Geometry: final body of the model. Coordinates: model frame, mm. Face numbers are marked on the shaded views. A direction names the side the tool comes from. Give positions to 0.01 mm unless a question says otherwise; leave off trailing zeros. Write each loop counter-clockwise with the first axis right and the second up, starting at its lowest first coordinate (ties: lowest second). Pieces come first, ordered by that corner, then holes.
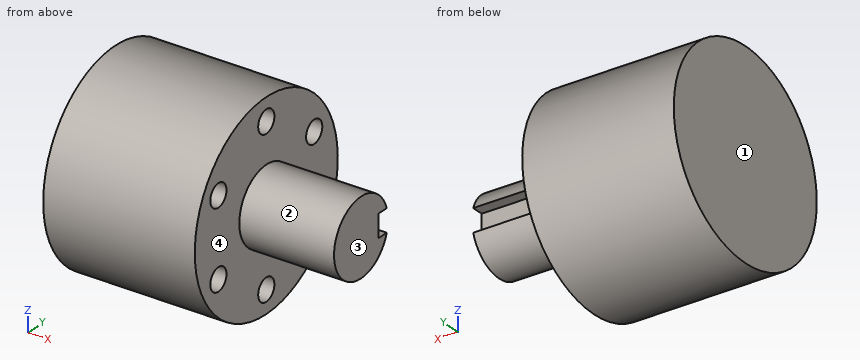
from build123d import *

# Parameters (mm, degrees)
SKETCH_1_R          = 13.25
EXTRUDE_1_DEPTH     = 20
SKETCH_2_R          = 1.5
CUT_EXTRUDE_1_DEPTH = 5
SKETCH_3_R          = 5
EXTRUDE_2_DEPTH     = 12.5
CUT_EXTRUDE_START   = -10
CUT_EXTRUDE_2_DEPTH = 10


with BuildPart() as part:
    # 草图1 → 凸台-拉伸1 (new body)
    with BuildSketch(Plane(origin=(0, 0, 0), x_dir=(0, 0, -1), z_dir=(1, 0, 0))):
        Circle(SKETCH_1_R)
    extrude(amount=EXTRUDE_1_DEPTH)

    # 草图2 → 切除-拉伸1 (cut)
    with BuildSketch(Plane(origin=(20, 0, 0), x_dir=(0, 0, -1), z_dir=(1, 0, 0))):
        with Locations((10.25, 0)):
            Circle(SKETCH_2_R)
        with Locations((5.125, -8.876760389)):
            Circle(SKETCH_2_R)
        with Locations((-5.125, -8.876760389)):
            Circle(SKETCH_2_R)
        with Locations((-10.25, 0)):
            Circle(SKETCH_2_R)
        with Locations((-5.125, 8.876760389)):
            Circle(SKETCH_2_R)
        with Locations((5.125, 8.876760389)):
            Circle(SKETCH_2_R)
    extrude(amount=-CUT_EXTRUDE_1_DEPTH, mode=Mode.SUBTRACT)

    # 草图3 → 凸台-拉伸2 (add)
    with BuildSketch(Plane(origin=(20, 0, 0), x_dir=(0, 0, -1), z_dir=(1, 0, 0))):
        Circle(SKETCH_3_R)
    extrude(amount=EXTRUDE_2_DEPTH)

    # 草图4 → 切除-拉伸2 (cut)
    with BuildSketch(Plane(origin=(32.5, 0, 0), x_dir=(0, 0, -1), z_dir=(1, 0, 0)).offset(CUT_EXTRUDE_START)):
        with BuildLine():
            Line((-1.5, 3.2), (1.5, 3.2))
            Line((1.5, 3.2), (1.5, 4.769696007))
            ThreePointArc((1.5, 4.769696007), (0, 5), (-1.5, 4.769696007))
            Line((-1.5, 4.769696007), (-1.5, 3.2))
        make_face()
    extrude(amount=CUT_EXTRUDE_2_DEPTH, mode=Mode.SUBTRACT)


solid = part.part
Q1. Section C-C on x = 30. Output: boundary loops of the cut face in (y, z), plus the area to 3 significant figures.
Filled sheet:
outline: (3.2, -1.5) - (3.2, 1.5) - (4.77, 1.5) arc R5 ccw (long way) to (4.77, -1.5) - close
area: 73.4 mm2
Q2. Pull-direction query (Y, two-part tool) for the marked faces 1 and 2; classes: released by +Y, released by -Y, zero draft, split by the parting line, or undercut.
Filled sheet:
face 1: zero draft
face 2: split by the parting line
Q3. Ray query, line 1 along X through (y, z) = (-6.75, -10.5); line 2 along Y through (x, z) = (5.5, 0.5); line 3 along Y through (x, z) = (18, 9.5). Return the intervals inside material, ascending.
Filled sheet:
line 1: x = 0 to 20
line 2: y = -13.24 to 13.24
line 3: y = -9.24 to -1.3, 1.3 to 9.24
Q4. Section B-B on y = 0. Output: boundary loops of the cut face in (x, z), plus the area to 3 significant figures.
Filled sheet:
outline: (0, -13.25) - (20, -13.25) - (20, -11.75) - (15, -11.75) - (15, -8.75) - (20, -8.75) - (20, -5) - (32.5, -5) - (32.5, 5) - (20, 5) - (20, 8.75) - (15, 8.75) - (15, 11.75) - (20, 11.75) - (20, 13.25) - (0, 13.25) - close
area: 625 mm2
Q5. Access query for the marked faces 3 and 4. Directions: +Z, -Z, +X, -X, +Y, -Y. A direction counts if a zero-diameter tool reaches every point of the face in a straight line with its end or side. Return the directions, or none.
Filled sheet:
face 3: +Z, -Z, +X, +Y, -Y
face 4: +X
Q6. Section D-D on z = 6. Output: boundary loops of the cut face in (x, y).
Filled sheet:
outline: (0, -11.81) - (20, -11.81) - (20, -10.1) - (15, -10.1) - (15, -7.66) - (20, -7.66) - (20, 7.66) - (15, 7.66) - (15, 10.1) - (20, 10.1) - (20, 11.81) - (0, 11.81) - close
Q7. Section A-A on z = 0. Output: boundary loops of the cut face in (x, y).
Filled sheet:
outline: (0, -13.25) - (20, -13.25) - (20, -5) - (32.5, -5) - (32.5, 3.2) - (22.5, 3.2) - (22.5, 5) - (20, 5) - (20, 13.25) - (0, 13.25) - close
Q8. Pin query (flat end, axial travel): P1, Ø1, axis at x = 11, z = -1, coming from the +Y side; P2, Ø2.5, axis at y = -9, z = 5, coming from the +X side; P3, Ø6, axis at x = 21, y = -6.5, coming from the -Z side. Return the tip coordinate at first contact, or that it passes through.
Filled sheet:
P1: stops at y = 13.24
P2: stops at x = 15
P3: stops at z = -12.73
